from build123d import *

# Parameters (mm, degrees)
AUFSATZ_LINEAR_AUSTRAGEN1_DEPTH = 125
SKIZZE2_R                       = 3.5
SCHNITT_LINEAR_AUSTRAGEN1_DEPTH = 60


with BuildPart() as part:
    # Skizze1 → Aufsatz-Linear austragen1 (new, symmetric)
    with BuildSketch(Plane.XY):
        with BuildLine():
            Line((-9, 15), (9, 15))
            ThreePointArc((9, 15), (13.242640687, 13.242640687), (15, 9))
            Line((15, 9), (15, -9))
            ThreePointArc((15, -9), (13.242640687, -13.242640687), (9, -15))
            Line((9, -15), (-9, -15))
            ThreePointArc((-9, -15), (-13.242640687, -13.242640687), (-15, -9))
            Line((-15, -9), (-15, 9))
            ThreePointArc((-15, 9), (-13.242640687, 13.242640687), (-9, 15))
        make_face()
        with BuildLine():
            Line((-13, 9), (-13, -9))
            ThreePointArc((-13, -9), (-11.828427125, -11.828427125), (-9, -13))
            Line((-9, -13), (9, -13))
            ThreePointArc((9, -13), (11.828427125, -11.828427125), (13, -9))
            Line((13, -9), (13, 9))
            ThreePointArc((13, 9), (11.828427125, 11.828427125), (9, 13))
            Line((9, 13), (-9, 13))
            ThreePointArc((-9, 13), (-11.828427125, 11.828427125), (-13, 9))
        make_face(mode=Mode.SUBTRACT)
    extrude(amount=AUFSATZ_LINEAR_AUSTRAGEN1_DEPTH, both=True)

    # Skizze2 → Schnitt-Linear austragen1 (cut)
    with BuildSketch(Plane(origin=(0, 15, 0), x_dir=(1, 0, 0), z_dir=(0, 1, 0))):
        with Locations(Location((0, 105, 0), (0, 0, 270))):
            Circle(SKIZZE2_R)
        with Locations(Location((0, 35, 0), (0, 0, 270))):
            Circle(SKIZZE2_R)
        with Locations((0, -35)):
            Circle(SKIZZE2_R)
        with Locations((0, -105)):
            Circle(SKIZZE2_R)
    extrude(amount=-SCHNITT_LINEAR_AUSTRAGEN1_DEPTH, mode=Mode.SUBTRACT)


solid = part.part
Can you work these out from the model? Positions are in its coordinate system, mm. A direction names the side the tool comes from. Give positions to 0.01 mm unless a question says otherwise; leave off trailing zeros. Loops run counter-clockwise (first coordinate to the right, second up) from the corner with the lowest first, then second, coordinate; pieces in that order, holes last. Notation, with made-up numbers: (7.25, 18) - (22.25, 18) arc R17 ccw to (22.25, 50) - close; hole circle Ø7 at (58, 7.5). An arc over 180 degrees is marked (long way). Return JSON: item names as keys, results as strings.
1. If I drill on line 1 (X direction, y = -5.75, z = -113); line 2 (Y direction, x = 12, z = -69), over which ranges is the centre line in solid material (lowest first)?
Output values:
{"line 1": "x = -15 to -13, 13 to 15", "line 2": "y = -14.2 to -11.65, 11.65 to 14.2"}
2. I want a section at B-B on y = -3. Please give me the cut outline in (x, z).
Output values:
{"outline": "(-15, -125) - (-13, -125) - (-13, 125) - (-15, 125) - close; (13, -125) - (15, -125) - (15, 125) - (13, 125) - close"}
3. We'd pull the mould along Z, two halves only. Please class faces 3 (the face through (-0.46, 14.01, 31.53)), 4 (the face through (13.4, 0.1, 125)), 5 (the face through (13.196, 13.289, 1.75)), 6 (the face through (-0.759, 14.014, 108.417)): +Z half, -Z half, draft (parallel to the pull), parting line (faces both ways), or undercut.
Output values:
{"face 3": "undercut", "face 4": "+Z half", "face 5": "draft", "face 6": "undercut"}
4. For faces 1 (the face through (-0.46, -13.99, 31.53)), 2 (the face through (11.797, -11.859, 1.75)), which set-ups out of +Z, -Z, +X, -X, +Y, -Y let a thin tool reach every point of the face, with its end or its side?
Output values:
{"face 1": "+Y, -Y", "face 2": "+Z, -Z"}
5. I want a section at C-C on x = 0. Give the number of separate pieces and of enclosed holes in the cut face, and give its area (3 significant figures).
Output values:
{"separate pieces": "10", "enclosed holes": "0", "area": "888 mm²"}
6. I want a section at A-A on z = 35. Please give me the cut outline in (x, y), and give its area (3 significant figures).
Output values:
{"outline": "(-15, -9) arc R6 ccw to (-9, -15) - (-3.5, -15) - (-3.5, -13) - (-9, -13) arc R4 cw to (-13, -9) - (-13, 9) arc R4 cw to (-9, 13) - (-3.5, 13) - (-3.5, 15) - (-9, 15) arc R6 ccw to (-15, 9) - close; (3.5, -15) - (9, -15) arc R6 ccw to (15, -9) - (15, 9) arc R6 ccw to (9, 15) - (3.5, 15) - (3.5, 13) - (9, 13) arc R4 cw to (13, 9) - (13, -9) arc R4 cw to (9, -13) - (3.5, -13) - close", "area": "179 mm²"}
